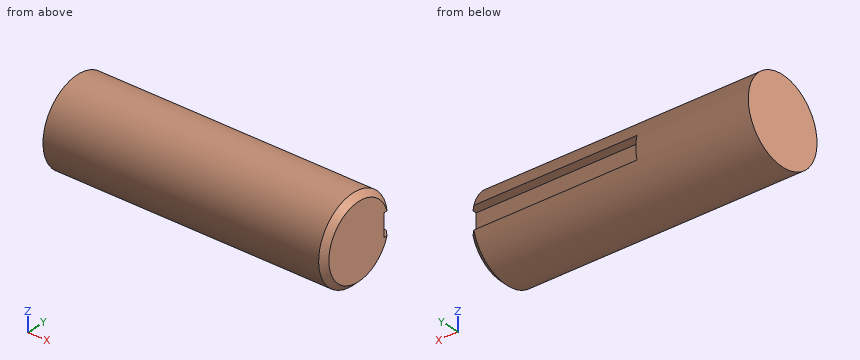
from build123d import *

# Parameters (mm, degrees)
SKETCH1_R           = 15
BOSS_EXTRUDE1_DEPTH = 50
CUT_EXTRUDE1_DEPTH  = 60
CHAMFER1_SIZE       = 2


with BuildPart() as part:
    # Sketch1 → Boss-Extrude1 (new, symmetric)
    with BuildSketch(Plane(origin=(0, 0, 0), x_dir=(0, 0, -1), z_dir=(1, 0, 0))):
        Circle(SKETCH1_R)
    extrude(amount=BOSS_EXTRUDE1_DEPTH, both=True)

    # Sketch2 → Cut-Extrude1 (cut)
    with BuildSketch(Plane(origin=(50, 0, 0), x_dir=(0, 0, -1), z_dir=(1, 0, 0))):
        Polygon((-4, 94.562608629), (-4, 14.456832295), (-4, 11), (4, 11), (4, 14.456832295), (4, 94.562608629), (4, 254.774161296), (-4, 254.774161296), align=None)
    extrude(amount=-CUT_EXTRUDE1_DEPTH, mode=Mode.SUBTRACT)

    # Chamfer1
    chamfer1_edges = [part.edges().sort_by_distance(p)[0] for p in [
        (50, -11.937336386, 9.082951062),
    ]]
    chamfer(chamfer1_edges, length=CHAMFER1_SIZE)


solid = part.part
Verification items for the finished model (mm, model axes). Coordinates: 2 decimals unless noted, no trailing zeros. Order: outer loops, then holes, each group sorted by start corner. A loop starts at its lowest first (then second) coordinate and runs counter-clockwise, first axis right, second up. Notation, with made-up numbers: (12.5, -21.75) -> (19.5, -21.75) arc R21 ccw to (19.5, 12.25) -> close; hole circle Ø5 at (19, 11.5). An arc over 180 degrees is marked (long way). Use CSV: the item, a comma, the result in double quotes. Start each with the question number.
Q1. Section check B-B, the plane x = -28.5. Record the cut outline in (y, z), and give its area (3 significant figures).
Q2. Section check C-C, the plane x = -9. Record the cut outline in (y, z).
Q3. Thickness scan on line 1 along Y through (x, z) = (1.5, -7.5); line 2 along Z through (x, y) = (3.5, -0.25); line 3 along X through (y, z) = (13.25, -0.75). Record the ranges inside material, lowest first.
Q4. Section check A-A, the plane z = 0. Record the cut outline in (x, y), and give its area (3 significant figures).
Q5. Depth check by flat-ended pin: P1, Ø1.7, axis at x = 24.5, y = 13.5, coming from the +Z side; P2, Ø4, axis at x = 34.5, y = 7, coming from the -Z side; P3, Ø2, axis at x = -19.5, y = 11, coming from the -Z side; P4, Ø12, axis at x = 12.5, y = 2, coming from the -Z side. Enter the tip coordinate at first touch or a pass-through.
Returned:
1,outline,"circle Ø30 at (0, 0)"
1,area,"707 mm^2"
2,outline,"(11, -4) -> (11, 4) -> (14.46, 4) arc R15 ccw (long way) to (14.46, -4) -> close"
3,line 1,"y = -12.99 to 12.99"
3,line 2,"z = -15 to 15"
3,line 3,"x = -50 to -10"
4,outline,"(-50, -15) -> (48, -15) -> (50, -13) -> (50, 11) -> (-10, 11) -> (-10, 15) -> (-50, 15) -> close"
4,area,"2,760 mm^2"
5,P1,"stops at z = 8.06"
5,P2,"stops at z = -14.14"
5,P3,"stops at z = -11.18"
5,P4,"stops at z = -15"
